Geometry: final body of the model. Coordinates: model frame, mm. A direction names the side the tool comes from. Round coordinates to 2 decimals unless told otherwise and drop trailing zeros. Loops run counter-clockwise (first coordinate to the right, second up) from the corner with the lowest first, then second, coordinate; pieces in that order, holes last. Notation, with made-up numbers: (82, 6.25) - (132, 6.25) arc R10 cw to (132, 12.25) - close; hole circle Ø5 at (68.25, -31). An arc over 180 degrees is marked (long way). Answer as a JSON object with one key per item and string values. Group by question number.
Item 1: First-contact query: pin 1 (20 mm diameter, centred on x = 4, y = -17, fed in from +Z); pin 2 (2 mm diameter, centred on y = 34, z = 1.5, fed in from -X); pin 3 (4 mm diameter, centred on y = 22, z = 3, fed in from +X); pin 4 (1.5 mm diameter, centred on x = 54.5, y = -0.5, fed in from +Z). Flat tips, straight axial feed; report the tip coordinate or a pass-through.
Item 2: Section B-B (x = -80). Return the cut outline in (y, z).
Item 3: Reachability of faces 4 (the face through (0, -7.8, 6)), 5 (the face through (-105, 0, 4)), 6 (the face through (-1, -45, 4)) from +Z, -Z, +X, -X, +Y, -Y: full face, straight path, thin tool, end or side. Return the list, or none.
Item 4: Line query: line 1 (Y direction, x = 27, z = 6.25); line 2 (X direction, y = 2, z = 4); line 3 (X direction, y = -19, z = 7.25). Output: solid intervals per line, ascending.
Item 5: Section C-C (y = 26). Return the cut outline in (x, z).
Item 6: Section A-A (z = 7.5). Return the cut outline in (x, y).
Item 7: Draft query along Z for faces 1 (the face through (0, -36, 6)), 2 (the face through (-1, 0, 3)), 3 (the face through (144.99, -0.99, 4.44)). Return one class per face: released by +Z, released by -Z, zero draft, split by the parting line, or undercut.
```python
from build123d import *

# Parameters (mm, degrees)
PAD_DEPTH       = 3
PAD001_DEPTH    = 3
SKETCH002_W     = 209.08447
SKETCH002_H     = 4.18
PAD002_DEPTH    = 3
SKETCH003_W     = 26.3
SKETCH003_H     = 34.2
POCKET_DEPTH    = 3
SKETCH004_W     = 18
SKETCH004_H     = 25
POCKET001_DEPTH = 3


with BuildPart() as part:
    # Sketch → Pad (new body)
    with BuildSketch(Plane.XY):
        with BuildLine():
            ThreePointArc((-100, 45), (-145, 0), (-100, -45))
            Line((-100, -45), (100, -45))
            ThreePointArc((100, -45), (145, 0), (100, 45))
            Line((-100, 45), (100, 45))
        make_face()
    extrude(amount=PAD_DEPTH)

    # Sketch001 (on Face6 of Pad) → Pad001 (join)
    with BuildSketch(Plane.XY.offset(3)):
        with BuildLine():
            ThreePointArc((-100, 45), (-145, 0), (-100, -45))
            Line((-100, -45), (100, -45))
            ThreePointArc((100, -45), (145, 0), (100, 45))
            Line((-100, 45), (100, 45))
        make_face()
        with BuildLine():
            ThreePointArc((-100, 5), (-105, 0), (-100, -5))
            Line((-100, -5), (100, -5))
            ThreePointArc((100, -5), (105, 0), (100, 5))
            Line((-100, 5), (100, 5))
        make_face(mode=Mode.SUBTRACT)
    extrude(amount=PAD001_DEPTH)

    # Sketch002 (on Face9 of Pad001) → Pad002 (join)
    with BuildSketch(Plane.XY.offset(6)):
        with BuildLine():
            ThreePointArc((-100, 45), (-145, 0), (-100, -45))
            Line((-100, -45), (100, -45))
            ThreePointArc((100, -45), (145, 0), (100, 45))
            Line((-100, 45), (100, 45))
        make_face()
        Rectangle(SKETCH002_W, SKETCH002_H, mode=Mode.SUBTRACT)
    extrude(amount=PAD002_DEPTH)

    # Sketch003 (on Face13 of Pad002) → Pocket (cut)
    with BuildSketch(Plane.XY.offset(9)):
        with Locations((0, -24.9)):
            Rectangle(SKETCH003_W, SKETCH003_H)
    extrude(amount=-POCKET_DEPTH, mode=Mode.SUBTRACT)

    # Sketch004 (on Face27 of Pocket) → Pocket001 (cut)
    with BuildSketch(Plane.XY.offset(6)):
        with Locations((0, -20.3)):
            Rectangle(SKETCH004_W, SKETCH004_H)
    extrude(amount=-POCKET001_DEPTH, mode=Mode.SUBTRACT)


solid = part.part
```
Values:
{
 "1": {"pin 1": "stops at z = 9", "pin 2": "stops at x = -130.59", "pin 3": "stops at x = 140.31", "pin 4": "stops at z = 3"},
 "2": {"outline": "(-45, 0) - (45, 0) - (45, 9) - (2.09, 9) - (2.09, 6) - (5, 6) - (5, 3) - (-5, 3) - (-5, 6) - (-2.09, 6) - (-2.09, 9) - (-45, 9) - close"},
 "3": {"face 4": "+Z", "face 5": "none", "face 6": "+Z, -Z, +X, -X, -Y"},
 "4": {"line 1": "y = -45 to -2.09, 2.09 to 45", "line 2": "x = -144.96 to -104.58, 104.58 to 144.96", "line 3": "x = -140.79 to -13.15, 13.15 to 140.79"},
 "5": {"outline": "(-136.73, 0) - (136.73, 0) - (136.73, 9) - (-136.73, 9) - close"},
 "6": {"outline": "(-100, -45) - (100, -45) arc R45 ccw to (100, 45) - (-100, 45) arc R45 ccw to start; hole (-104.54, -2.09) - (104.54, -2.09) - (104.54, 2.09) - (-104.54, 2.09) - close; hole (-13.15, -42) - (13.15, -42) - (13.15, -7.8) - (-13.15, -7.8) - close"},
 "7": {"face 1": "released by +Z", "face 2": "undercut", "face 3": "zero draft"}
}
